Model file for the job. Use its own axes, mm. Face numbers are marked on the shaded views. A direction names the side the tool comes from. Coordinates: 2 decimals unless noted, no trailing zeros. Order: outer loops, then holes, each group sorted by start corner. A loop starts at its lowest first (then second) coordinate and runs counter-clockwise, first axis right, second up. Notation, with made-up numbers: M -23,-31.5 L -6,-31.5 A14 ccw -6,-19.5 Z; hole C 63,74.25 d9. An arc over 180 degrees is marked long. Return JSON: item names as keys, results as strings.
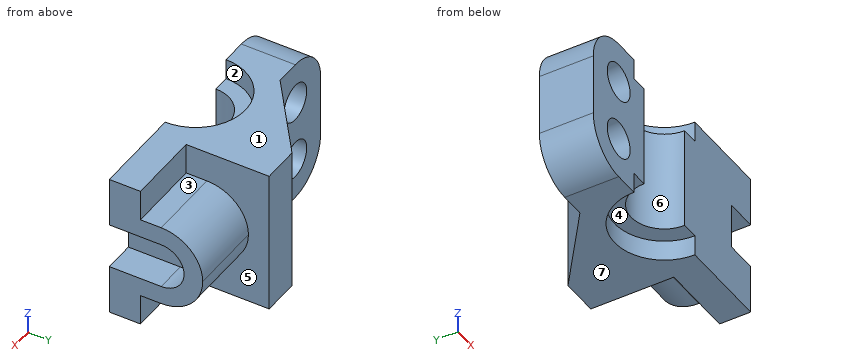
```python
from build123d import *

# Parameters (mm, degrees)
EXTRUDE_1_DEPTH     = 70
FILLET_1_R          = 20
SKETCH_4_R          = 9
CUT_EXTRUDE_1_DEPTH = 146.316895095
CUT_EXTRUDE_2_DEPTH = 10
CUT_EXTRUDE_3_DEPTH = 153.646650799
CUT_EXTRUDE_START   = -10
SKETCH_6_R          = 24
CUT_EXTRUDE_4_DEPTH = 10
EXTRUDE_2_DEPTH     = 36
CUT_EXTRUDE_5_DEPTH = 15


with BuildPart() as part:
    # Sketch 3 → Extrude 1 (new body)
    with BuildSketch(Plane.XY):
        Polygon((0, 0), (0, 26), (32, 26), (70, 55), (88, 55), (88, 15), (124, 15), (124, 0), (30.697426797, 0), align=None)
    extrude(amount=-EXTRUDE_1_DEPTH)

    # Fillet 1
    fillet_1_edges = [part.edges().sort_by_distance(p)[0] for p in [
        (0, 13, -70),
        (0, 13, 0),
    ]]
    fillet(fillet_1_edges, radius=FILLET_1_R)

    # Sketch 4 → Cut-Extrude 1 (cut, through all)
    with BuildSketch(Plane(origin=(0, 26, 0), x_dir=(1, 0, 0), z_dir=(0, 1, 0))):
        with Locations(Location((20, 20, 0), (0, 0, 270))):
            Circle(SKETCH_4_R)
        with Locations(Location((20, 50, 0), (0, 0, 270))):
            Circle(SKETCH_4_R)
    extrude(amount=-CUT_EXTRUDE_1_DEPTH, mode=Mode.SUBTRACT)

    # Sketch 5 → Cut-Extrude 2 (cut)
    with BuildSketch(Plane.XY):
        with BuildLine():
            ThreePointArc((80, 0), (56, 24), (32, 0))
            Line((32, 0), (40, 0))
            ThreePointArc((40, 0), (56, 16), (72, 0))
            Line((72, 0), (80, 0))
        make_face()
    extrude(amount=-CUT_EXTRUDE_2_DEPTH, mode=Mode.SUBTRACT)

    # Sketch 5_3 → Cut-Extrude 3 (cut, through all)
    with BuildSketch(Plane.XY):
        with BuildLine():
            ThreePointArc((72, 0), (56, 16), (40, 0))
            Line((40, 0), (72, 0))
        make_face()
    extrude(amount=-CUT_EXTRUDE_3_DEPTH, mode=Mode.SUBTRACT)

    # Sketch 6 → Cut-Extrude 4 (cut)
    with BuildSketch(Plane(origin=(0, 0, -70), x_dir=(-1, 0, 0), z_dir=(0, 0, -1)).offset(CUT_EXTRUDE_START)):
        with Locations((-56, 0)):
            Circle(SKETCH_6_R)
    extrude(amount=CUT_EXTRUDE_4_DEPTH, mode=Mode.SUBTRACT)

    # Sketch 7 → Extrude 2 (add)
    with BuildSketch(Plane(origin=(88, 0, 0), x_dir=(0, 0, -1), z_dir=(1, 0, 0))):
        with BuildLine():
            Line((35, 45), (35, 15))
            Line((35, 15), (55, 15))
            Line((55, 15), (55, 25))
            ThreePointArc((55, 25), (49.142135624, 39.142135624), (35, 45))
        make_face()
        with BuildLine():
            Line((15, 15), (35, 15))
            Line((35, 15), (35, 45))
            ThreePointArc((35, 45), (20.857864376, 39.142135624), (15, 25))
            Line((15, 25), (15, 15))
        make_face()
    extrude(amount=EXTRUDE_2_DEPTH)

    # Sketch 8 → Cut-Extrude 5 (cut)
    with BuildSketch(Plane(origin=(124, 0, 0), x_dir=(0, 0, -1), z_dir=(1, 0, 0))):
        with BuildLine():
            Line((24, 0), (24, 25))
            ThreePointArc((24, 25), (35, 36), (46, 25))
            Line((46, 25), (46, 0))
            Line((46, 0), (24, 0))
        make_face()
    extrude(amount=-CUT_EXTRUDE_5_DEPTH, mode=Mode.SUBTRACT)


solid = part.part
```
Item 1: Drop flat-ended pins along their axis: pin 1 Ø6 at (x, y) = (99.5, 39.5) entering from -Z; pin 2 Ø2 at (y, z) = (44, -51) entering from +X; pin 3 Ø4.5 at (x, z) = (110, -10.5) entering from +Y. Give the stop position or say it passes through.
Check result:
{"pin 1": "stops at z = -51.36", "pin 2": "stops at x = 88", "pin 3": "stops at y = 15"}
Item 2: Pull direction X, two halves, no side cores. Call the marked faces 5, 6 and 7: +X half, -X half, draft (parallel to the pull), parting line (faces both ways), or undercut.
Check result:
{"face 5": "+X half", "face 6": "undercut", "face 7": "draft"}
Item 3: Saw through at B-B (x = 18). Write the cut outline in (y, z).
Check result:
{"outline": "M 0,-69.9 L 26,-69.9 L 26,-58.77 L 0,-58.77 Z; M 0,-41.23 L 26,-41.23 L 26,-28.77 L 0,-28.77 Z; M 0,-11.23 L 26,-11.23 L 26,-0.1 L 0,-0.1 Z"}
Item 4: Saw through at D-D (y = 5). Write the cut outline in (x, z).
Check result:
{"outline": "M 0,-50 A20 ccw 20,-70 L 32.53,-70 L 32.53,-60 L 40.8,-60 L 40.8,-10 L 32.53,-10 L 32.53,0 L 20,0 A20 ccw 0,-20 Z; M 71.2,-60 L 79.47,-60 L 79.47,-70 L 124,-70 L 124,-46 L 109,-46 L 109,-24 L 124,-24 L 124,0 L 79.47,0 L 79.47,-10 L 71.2,-10 Z; hole C 20,-50 d18; hole C 20,-20 d18"}
Item 5: Wall check: line 1 (X direction, y = 5.5, z = -19); line 2 (X direction, y = 6.25, z = -50); line 3 (Y direction, x = 10, z = -20.5). Give the ranges that are in metal, low to high.
Check result:
{"line 1": "x = 0.03 to 11.06, 28.94 to 40.98, 71.02 to 124", "line 2": "x = 0 to 11, 29 to 41.27, 70.73 to 124", "line 3": "y = 0 to 26"}
Item 6: Saw through at C-C (x = 102.5). Write the cut outline in (y, z).
Check result:
{"outline": "M 0,-70 L 15,-70 L 15,-55 L 25,-55 A20 ccw 25,-15 L 15,-15 L 15,0 L 0,0 Z"}
Item 7: Saw through at A-A (y = 13.5). Write the cut outline in (x, z).
Check result:
{"outline": "M 0,-50 A20 ccw 20,-70 L 36.16,-70 L 36.16,-60 L 47.41,-60 L 47.41,-10 L 36.16,-10 L 36.16,0 L 20,0 A20 ccw 0,-20 Z; M 64.59,-60 L 75.84,-60 L 75.84,-70 L 124,-70 L 124,-46 L 109,-46 L 109,-24 L 124,-24 L 124,0 L 75.84,0 L 75.84,-10 L 64.59,-10 Z; hole C 20,-50 d18; hole C 20,-20 d18"}
Item 8: 3-axis set-ups, long thin cutter, end or side, ignore diameter. For the marked faces 1, 2, 3 and 4: which of +Z, -Z, +X, -X, +Y, -Y reach the whole face in a straight line?
Check result:
{"face 1": "+Z, +X, -X, +Y, -Y", "face 2": "+Z, -Y", "face 3": "+Z, +X, +Y", "face 4": "-Z, -Y"}
